from build123d import *

# Parameters (mm, degrees)
F0_R     = 3.5
F1_DEPTH = 20
F2_R     = 25
F3_DEPTH = 2
F4_R     = 5.17
F5_DEPTH = 4
F6_R     = 2.5
F7_DEPTH = 2


with BuildPart() as f1:
    # F0 (on Top) → F1 (new body)
    with BuildSketch(Plane.XY):
        Circle(F0_R)
    extrude(amount=-F1_DEPTH)

    # F2 (on Top) → F3 (join)
    with BuildSketch(Plane.XY):
        Circle(F2_R)
    extrude(amount=F3_DEPTH)

    # F4 (on Top) → F5 (join)
    with BuildSketch(Plane.XY):
        with Locations((-20.68, 0)):
            Circle(F4_R)
        with Locations((-10.34, -17.909405)):
            Circle(F4_R)
        with Locations((10.34, -17.909405)):
            Circle(F4_R)
        with Locations((20.68, 0)):
            Circle(F4_R)
        with Locations((10.34, 17.909405)):
            Circle(F4_R)
        with Locations((-10.34, 17.909405)):
            Circle(F4_R)
    extrude(amount=F5_DEPTH)

    # F6 (on face) → F7 (join)
    with BuildSketch(Plane.XY.offset(2)):
        with BuildLine():
            Line((-5, 40), (-5, 0))
            Line((-5, 0), (5, 0))
            Line((5, 0), (5, 40))
            ThreePointArc((5, 40), (0, 45), (-5, 40))
        make_face()
        with Locations((0, 40)):
            Circle(F6_R, mode=Mode.SUBTRACT)
    extrude(amount=-F7_DEPTH)


solid = f1.part
Verification items for the finished model (mm, model axes). A direction names the side the tool comes from. Give positions to 0.01 mm unless a question says otherwise; leave off trailing zeros. Write each loop counter-clockwise with the first axis right and the second up, starting at its lowest first coordinate (ties: lowest second). Pieces come first, ordered by that corner, then holes.
(1) Access from +Z, -Z, +X, -X, +Y, -Y to the whole of each face (thin tool, end or side, straight path). Record for faces 4 (the face through (3.233, -1.341, -9.86)), 5 (the face through (-5, 32, 1)), 6 (the face through (13.12, 22.27, 2.86)), 7 (the face through (-21.72, -12.38, 0.99)).
(2) Cross-section at A-A (x = 0). Enter the section's corners in (y, z), plus the area to 3 significant figures.
(3) Mould release check, pull along Y, two halves, no side actions. Record for faces 1 (the face through (-11.461, -22.956, 2.861)), 2 (the face through (-7, 24, 1)), 3 (the face through (21, 0, 4)): +Y half, -Y half, draft (parallel to the pull), parting line (faces both ways), or undercut.
(4) Cross-section at C-C (x = 19). Enter the section's corners in (y, z).
(5) Cross-section at D-D (z = -10.25). Enter the section's corners in (x, y), plus the area to 3 significant figures.
(6) Material ranges on line 1 (Y direction, x = 0, z = 1.55); line 2 (Z direction, x = 12.5, y = 0.5); line 3 (Z direction, x = 11.5, y = -15), recorded low to high.
(7) Cross-section at B-B (y = 0). Enter the section's corners in (x, z), plus the area to 3 significant figures.
(8) Gauge pin test, flat ends, axial feed: pin 1 (1 mm diameter, centred on y = 32.5, z = 1.5, fed in from +X); pin 2 (3 mm diameter, centred on x = 9, z = -0.5, fed in from -Y); pin 3 (6 mm diameter, centred on x = -9.5, y = -3.5, fed in from -Z). Record the tip position at first contact, or that the pin passes through.
Worked out:
1. face 4: -Z
1. face 5: +Z, -Z, -X, +Y
1. face 6: +Z
1. face 7: +Z, -Z, -X, -Y
2. outline: (-25, 0) - (-3.5, 0) - (-3.5, -20) - (3.5, -20) - (3.5, 0) - (37.5, 0) - (37.5, 2) - (-25, 2) - close; (42.5, 0) - (45, 0) - (45, 2) - (42.5, 2) - close
2. area: 270 mm2
3. face 1: undercut
3. face 2: +Y half
3. face 3: draft
4. outline: (-16.25, 0) - (16.25, 0) - (16.25, 2) - (4.89, 2) - (4.89, 4) - (-4.89, 4) - (-4.89, 2) - (-16.25, 2) - close
5. outline: circle Ø7 at (0, 0)
5. area: 38.5 mm2
6. line 1: y = -25 to 37.5, 42.5 to 45
6. line 2: z = 0 to 2
6. line 3: z = 0 to 4
7. outline: (-25.85, 0) - (-3.5, 0) - (-3.5, -20) - (3.5, -20) - (3.5, 0) - (25.85, 0) - (25.85, 4) - (15.51, 4) - (15.51, 2) - (-15.51, 2) - (-15.51, 4) - (-25.85, 4) - close
7. area: 285 mm2
8. pin 1: stops at x = 5
8. pin 2: stops at y = -23.82
8. pin 3: stops at z = 0
